Design review of the part built by this model. Coordinates are the model's own, in mm. A direction names the side the tool comes from. Coordinates: 2 decimals unless noted, no trailing zeros. Write each loop counter-clockwise with the first axis right and the second up, starting at its lowest first coordinate (ties: lowest second). Pieces come first, ordered by that corner, then holes. Notation, with made-up numbers: (82.25, -40) - (110.25, -40) arc R17 cw to (110.25, -36) - close; hole circle Ø7 at (2, -5.75). An arc over 180 degrees is marked (long way). Answer as a JSON object with one key per item and string values.
```python
from build123d import *

# Parameters (mm, degrees)
STOCK_NEW_TRACKER_1_OUTLINE_R  = 10.415
STOCK_NEW_TRACKER_1_DEPTH      = 10
FILLET1_R                      = 12.7
SKETCH6_R                      = 10.4
CUT_EXTRUDE5_DEPTH             = 243.280828936
CUT_EXTRUDE1_START             = -5
CUT_EXTRUDE1_DEPTH             = 5
SKETCH2_R                      = 10.415
SKETCH2_R_2                    = 4
BOSS_EXTRUDE1_DEPTH            = 5
SKETCH3_R                      = 5.15
CUT_EXTRUDE2_DEPTH             = 3
SKETCH4_R                      = 11.125
CUT_EXTRUDE3_DEPTH             = 2
SKETCH5_R                      = 1.25
CUT_EXTRUDE4_DEPTH             = 243.092957495
SKETCH7_R                      = 190
SKETCH7_R_2                    = 134
CUT_EXTRUDE6_DEPTH             = 243.126000399
M5_CLEARANCE_HOLE1_D           = 5.5
M5_CLEARANCE_HOLE1_DEPTH       = 7.5
M5_CLEARANCE_HOLE1_CSINK_D     = 5.55
M5_CLEARANCE_HOLE1_CSINK_ANGLE = 90
M5_CLEARANCE_HOLE1_TIP         = 1.652366702
M4_CLEARANCE_HOLE1_D           = 4.5
M4_CLEARANCE_HOLE1_DEPTH       = 7.5
M4_CLEARANCE_HOLE1_CSINK_D     = 4.55
M4_CLEARANCE_HOLE1_CSINK_ANGLE = 90
M4_CLEARANCE_HOLE1_TIP         = 1.351936393


# Read off the part's stored shape, not the designer's step: Stock-New_Tracker-1
with BuildPart() as part:
    # Stock-New_Tracker-1 outline → Stock-New_Tracker-1 (new body)
    with BuildSketch(Plane(origin=(0, 0, 0), x_dir=(1, 0, 0), z_dir=(0, 1, 0))):
        with BuildLine():
            ThreePointArc((144.666666667, 39.642849993), (-150, 0), (144.666666667, -39.642849993))
            ThreePointArc((144.666666667, -39.642849993), (190, 0), (144.666666667, 39.642849993))
        make_face()
        with Locations((168.805, 0)):
            Circle(STOCK_NEW_TRACKER_1_OUTLINE_R, mode=Mode.SUBTRACT)
    extrude(amount=STOCK_NEW_TRACKER_1_DEPTH)

    # Fillet1
    fillet1_edges = [part.edges().sort_by_distance(p)[0] for p in [
        (144.666666667, 5, 39.642849993),
        (144.666666667, 5, -39.642849993),
    ]]
    fillet(fillet1_edges, radius=FILLET1_R)

    # Sketch6 → Cut-Extrude5 (cut, through all)
    with BuildSketch(Plane.XZ):
        with Locations(Location((-115, 0, 0), (0, 0, 270))):
            Circle(SKETCH6_R)
    extrude(amount=-CUT_EXTRUDE5_DEPTH, mode=Mode.SUBTRACT)

    # Sketch1 → Cut-Extrude1 (cut)
    with BuildSketch(Plane(origin=(0, 10, 0), x_dir=(1, 0, 0), z_dir=(0, 1, 0)).offset(CUT_EXTRUDE1_START)):
        with BuildLine():
            ThreePointArc((153.020872865, -39.885765971), (190, 0), (153.020872865, 39.885765971))
            ThreePointArc((153.020872865, 39.885765971), (146.205916285, 42.506906245), (141.960663798, 48.447599878))
            ThreePointArc((141.960663798, 48.447599878), (-150, 0), (141.960663798, -48.447599878))
            ThreePointArc((141.960663798, -48.447599878), (146.205916285, -42.506906245), (153.020872865, -39.885765971))
        make_face()
    extrude(amount=CUT_EXTRUDE1_DEPTH, mode=Mode.SUBTRACT)

    # Sketch2 → Boss-Extrude1 (add)
    with BuildSketch(Plane.XZ):
        with Locations((-115, 0)):
            Circle(SKETCH2_R)
        with Locations(Location((-115, 0, 0), (0, 0, 270))):
            Circle(SKETCH2_R_2, mode=Mode.SUBTRACT)
    extrude(amount=-BOSS_EXTRUDE1_DEPTH)

    # Sketch3 → Cut-Extrude2 (cut)
    with BuildSketch(Plane(origin=(0, 5, 0), x_dir=(1, 0, 0), z_dir=(0, 1, 0))):
        with Locations(Location((-115, 0, 0), (0, 0, 270))):
            Circle(SKETCH3_R)
    extrude(amount=-CUT_EXTRUDE2_DEPTH, mode=Mode.SUBTRACT)

    # Sketch4 → Cut-Extrude3 (cut)
    with BuildSketch(Plane(origin=(0, 5, 0), x_dir=(1, 0, 0), z_dir=(0, 1, 0))):
        with Locations(Location((-115, 0, 0), (0, 0, 270))):
            Circle(SKETCH4_R)
    extrude(amount=-CUT_EXTRUDE3_DEPTH, mode=Mode.SUBTRACT)

    # Sketch5 → Cut-Extrude4 (cut, through all)
    with BuildSketch(Plane(origin=(0, 3, 0), x_dir=(1, 0, 0), z_dir=(0, 1, 0))):
        with Locations(Location((-118.5, -6.062177826, 0), (0, 0, 270))):
            Circle(SKETCH5_R)
        with Locations(Location((-118.5, 6.062177826, 0), (0, 0, 270))):
            Circle(SKETCH5_R)
        with Locations(Location((-108, 0, 0), (0, 0, 270))):
            Circle(SKETCH5_R)
    extrude(amount=-CUT_EXTRUDE4_DEPTH, mode=Mode.SUBTRACT)

    # Sketch7 → Cut-Extrude6 (cut, through all)
    with BuildSketch(Plane(origin=(0, 5, 0), x_dir=(1, 0, 0), z_dir=(0, 1, 0))):
        Circle(SKETCH7_R)
        with Locations(Location((0, 0, 0), (0, 0, 270))):
            Circle(SKETCH7_R_2, mode=Mode.SUBTRACT)
    extrude(amount=-CUT_EXTRUDE6_DEPTH, mode=Mode.SUBTRACT)

    # M5 Clearance Hole1
    with Locations(Plane(origin=(0, 5, 0), x_dir=(1, 0, 0), z_dir=(0, 1, 0))):
        with Locations((-65, 112.583302492), (130, 0), (-65, -112.583302492)):
            CounterSinkHole(M5_CLEARANCE_HOLE1_D / 2, M5_CLEARANCE_HOLE1_CSINK_D / 2, depth=M5_CLEARANCE_HOLE1_DEPTH, counter_sink_angle=M5_CLEARANCE_HOLE1_CSINK_ANGLE)
            with Locations((0, 0, -(M5_CLEARANCE_HOLE1_DEPTH + M5_CLEARANCE_HOLE1_TIP / 2))):  # 118° drill point
                Cone(0, M5_CLEARANCE_HOLE1_D / 2, M5_CLEARANCE_HOLE1_TIP, mode=Mode.SUBTRACT)

    # M4 Clearance Hole1
    with Locations(Plane(origin=(0, 5, 0), x_dir=(1, 0, 0), z_dir=(0, 1, 0))):
        with Locations((-70.875, -30), (-70.875, 0), (-70.875, 30), (70.875, -30), (70.875, 0), (70.875, 30)):
            CounterSinkHole(M4_CLEARANCE_HOLE1_D / 2, M4_CLEARANCE_HOLE1_CSINK_D / 2, depth=M4_CLEARANCE_HOLE1_DEPTH, counter_sink_angle=M4_CLEARANCE_HOLE1_CSINK_ANGLE)
            with Locations((0, 0, -(M4_CLEARANCE_HOLE1_DEPTH + M4_CLEARANCE_HOLE1_TIP / 2))):  # 118° drill point
                Cone(0, M4_CLEARANCE_HOLE1_D / 2, M4_CLEARANCE_HOLE1_TIP, mode=Mode.SUBTRACT)


solid = part.part
```
(1) To check wall thickness, follow line 1 (Z direction, x = -72, y = 2.85); line 2 (X direction, y = 0.8, z = -29.5); line 3 (X direction, y = 1.65, z = -2.5). State the ranges of each line that lie inside material, in increasing order. Write a range as from..to.
Solved:
{"line 1": "z = -113.01..-31.95, -28.05..-1.95, 1.95..28.05, 31.95..113.01", "line 2": "x = -130.71..-73.07, -68.68..68.68, 73.07..130.71", "line 3": "x = -133.98..-118.12, -111.88..128.85, 131.15..133.98"}
(2) Take a section at B-B, the plane z = 82. Write out the cut boundary in (x, y).
Solved:
{"outline": "(-105.98, 0) - (105.98, 0) - (105.98, 5) - (-105.98, 5) - close"}
(3) Take a section at A-A, the plane x = 40.5. Write out the cut boundary in (y, z), and give its area (3 significant figures).
Solved:
{"outline": "(0, -127.73) - (5, -127.73) - (5, 127.73) - (0, 127.73) - close", "area": "1,280 mm^2"}
(4) For pin 1 (6 mm diameter, centred on x = 47.5, z = 49, fed in from -Y); pin 2 (2 mm diameter, centred on y = 4, z = 57, fed in from +X); pin 3 (3 mm diameter, centred on x = -108, z = 0, fed in from +Y); pin 4 (3 mm diameter, centred on x = -42.5, y = 2.5, fed in from -Z), all flat-tipped, find the tip position at first contact; note any pin that passes through.
Solved:
{"pin 1": "stops at y = 0", "pin 2": "stops at x = 121.74", "pin 3": "stops at y = 3", "pin 4": "stops at z = -127.57"}
(5) Tool access review of faces 4 (the face through (-111.034, 0.986, 0.521)), 5 (the face through (-120, 3, 2)): name each direction out of +Z, -Z, +X, -X, +Y, -Y from which nothing blocks a thin tool from reaching the whole face with its end or side.
Solved:
{"face 4": "+Y, -Y", "face 5": "+Y"}
(6) The part is to be moulded in two halves that separate along X. For faces 1 (the face through (-2, 5, -2)), 2 (the face through (-118, 2, 3)), 3 (the face through (-118.9, 2.5, 61.8)), say which applies: pulls with the +X half, pulls with the -X half, needs draft (parallel to the pull), parting line crosses it, or undercut.
Solved:
{"face 1": "needs draft", "face 2": "undercut", "face 3": "parting line crosses it"}
